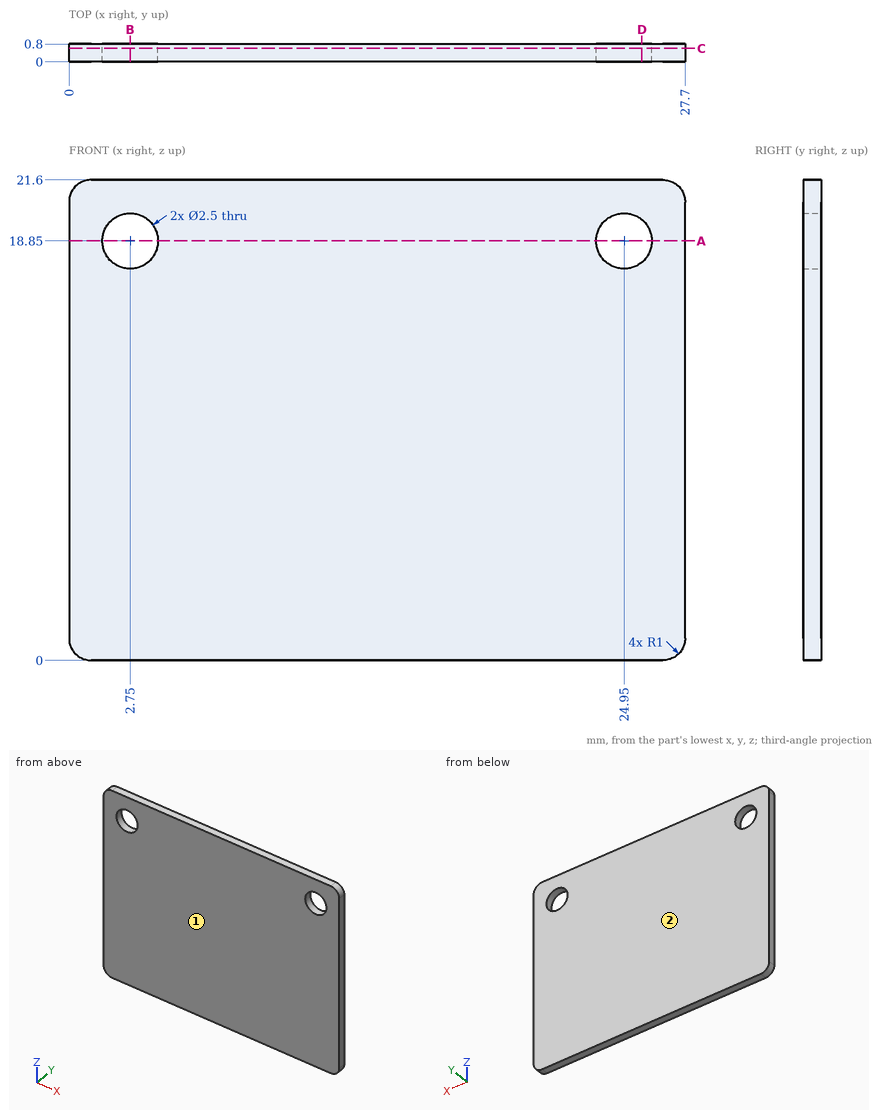
Job drawing, mm, ordinate dimensions from the low corner. One solid piece. Round coordinates to 2 decimals unless told otherwise and drop trailing zeros. Order: outer loops, then holes, each group sorted by start corner. A loop starts at its lowest first (then second) coordinate and runs counter-clockwise, first axis right, second up. Notation, with made-up numbers: (-24, 71) -> (34, 71) arc R16 ccw to (34, 82) -> close; hole circle Ø9 at (1.5, 74.5). An arc over 180 degrees is marked (long way). Answer in a Markdown table with one row per item.
1) Mould opens along Y. For the marked faces 1 and 2 say: released by +Y, released by -Y, zero draft, split by the parting line, or undercut.
Values:
| item | result |
|---|---|
| face 1 | released by -Y |
| face 2 | released by +Y |
2) Band-saw the part on D-D on x = 25.75. Give the cut face in (y, z).
Values:
| item | result |
|---|---|
| outline | (0, 0) -> (0.8, 0) -> (0.8, 17.89) -> (0, 17.89) -> close; (0, 19.81) -> (0.8, 19.81) -> (0.8, 21.6) -> (0, 21.6) -> close |
3) Wall check: L1, parallel to X at y = 0.3, z = 18.85; L2, parallel to Z at x = 24, y = 0.6. Give the ranges that are in metal, low to high.
Values:
| item | result |
|---|---|
| L1 | 0 to 1.5, 4 to 23.7, 26.2 to 27.7 |
| L2 | 0 to 18.04, 19.66 to 21.6 |
4) Band-saw the part on C-C on y = 0.6. Give the cut face in (x, z), and give its area (3 significant figures).
Values:
| item | result |
|---|---|
| outline | (0, 1) arc R1 ccw to (1, 0) -> (26.7, 0) arc R1 ccw to (27.7, 1) -> (27.7, 20.6) arc R1 ccw to (26.7, 21.6) -> (1, 21.6) arc R1 ccw to (0, 20.6) -> close; hole circle Ø2.5 at (2.75, 18.85); hole circle Ø2.5 at (24.95, 18.85) |
| area | 588 mm2 |
5) Band-saw the part on A-A on z = 18.85. Give the cut face in (x, y).
Values:
| item | result |
|---|---|
| outline | (0, 0) -> (1.5, 0) -> (1.5, 0.8) -> (0, 0.8) -> close; (4, 0) -> (23.7, 0) -> (23.7, 0.8) -> (4, 0.8) -> close; (26.2, 0) -> (27.7, 0) -> (27.7, 0.8) -> (26.2, 0.8) -> close |
6) Band-saw the part on B-B on x = 2.75. Give the cut face in (y, z), and give its area (3 significant figures).
Values:
| item | result |
|---|---|
| outline | (0, 0) -> (0.8, 0) -> (0.8, 17.6) -> (0, 17.6) -> close; (0, 20.1) -> (0.8, 20.1) -> (0.8, 21.6) -> (0, 21.6) -> close |
| area | 15.3 mm2 |
